Could you check a few things on this drawing? It's one solid part, dimensions in mm from its lowest x, y, z. A direction names the side the tool comes from. Round coordinates to 2 decimals unless told otherwise and drop trailing zeros. Write each loop counter-clockwise with the first axis right and the second up, starting at its lowest first coordinate (ties: lowest second). Pieces come first, ordered by that corner, then holes. Notation, with made-up numbers: (33.5, -24.75) -> (83.5, -24.75) arc R27 cw to (83.5, -2.75) -> close; hole circle Ø1 at (35, 57). An arc over 180 degrees is marked (long way). Return JSON: item names as keys, results as strings.
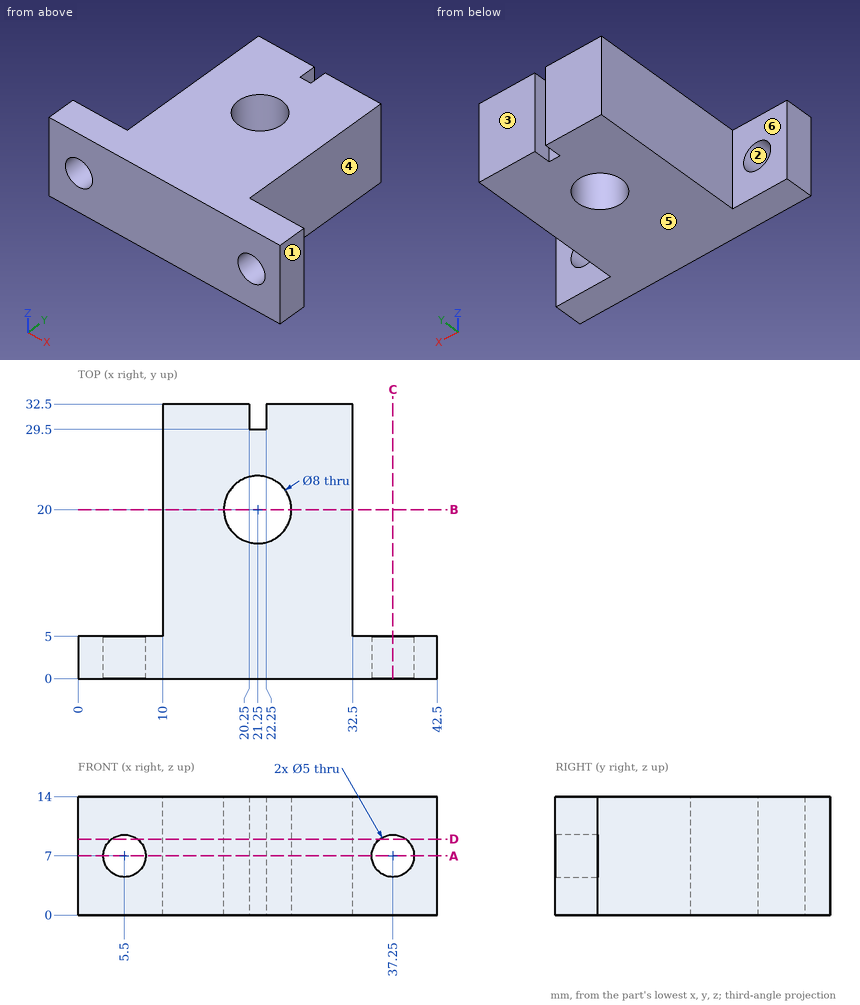
1) I want a section at A-A, the plane z = 7. Please give me the cut outline in (x, y), and give its area (3 significant figures).
Return value:
{"outline": "(0, 0) -> (3, 0) -> (3, 5) -> (0, 5) -> close; (8, 0) -> (34.75, 0) -> (34.75, 5) -> (32.5, 5) -> (32.5, 32.5) -> (22.25, 32.5) -> (22.25, 29.5) -> (20.25, 29.5) -> (20.25, 32.5) -> (10, 32.5) -> (10, 5) -> (8, 5) -> close; (39.75, 0) -> (42.5, 0) -> (42.5, 5) -> (39.75, 5) -> close; hole circle Ø8 at (21.25, 20)", "area": "725 mm²"}
2) Will these pins go through, and if not, where does the flat tip stop? pin 1 Ø3 at (y, z) = (21.5, 3) entering from -X; pin 2 Ø7 at (y, z) = (19.5, 7.5) entering from +X; pin 3 Ø5 at (x, z) = (4.5, 4.5) entering from +Y.
Return value:
{"pin 1": "x = 10", "pin 2": "x = 32.5", "pin 3": "y = 5"}
3) I want a section at D-D, the plane z = 9. Please give me the cut outline in (x, y).
Return value:
{"outline": "(0, 0) -> (4, 0) -> (4, 5) -> (0, 5) -> close; (7, 0) -> (35.75, 0) -> (35.75, 5) -> (32.5, 5) -> (32.5, 32.5) -> (22.25, 32.5) -> (22.25, 29.5) -> (20.25, 29.5) -> (20.25, 32.5) -> (10, 32.5) -> (10, 5) -> (7, 5) -> close; (38.75, 0) -> (42.5, 0) -> (42.5, 5) -> (38.75, 5) -> close; hole circle Ø8 at (21.25, 20)"}
4) I want a section at C-C, the plane x = 37.25. Please give me the cut outline in (y, z), and give its area (3 significant figures).
Return value:
{"outline": "(0, 0) -> (5, 0) -> (5, 4.5) -> (0, 4.5) -> close; (0, 9.5) -> (5, 9.5) -> (5, 14) -> (0, 14) -> close", "area": "45.0 mm²"}
5) Thinking about a two-plate mould opening in X: for the marked faces 1, 2 and 3, which applies, pulls with the +X half, pulls with the -X half, needs draft (parallel to the pull), parting line crosses it, or undercut?
Return value:
{"face 1": "pulls with the +X half", "face 2": "undercut", "face 3": "needs draft"}
6) For the marked faces 4, 5 and 6, which set-ups out of +Z, -Z, +X, -X, +Y, -Y let a thin tool reach every point of the face, with its end or its side?
Return value:
{"face 4": "+Z, -Z, +X, +Y", "face 5": "-Z, +X, -X, +Y, -Y", "face 6": "+Z, -Z, -X, +Y"}
7) I want a section at B-B, the plane y = 20. Please give me the cut outline in (x, z), and give its area (3 significant figures).
Return value:
{"outline": "(10, 0) -> (17.25, 0) -> (17.25, 14) -> (10, 14) -> close; (25.25, 0) -> (32.5, 0) -> (32.5, 14) -> (25.25, 14) -> close", "area": "203 mm²"}
8) If I drill on probe 1 along X at (y, z) = (31.5, 13); probe 2 along Y at (x, z) = (21.25, 8); probe 3 along Z at (x, y) = (37.25, 1.75), over which ranges is the centre line in solid material (lowest first)? Write a range as [from, to].
Return value:
{"probe 1": "[10, 20.25], [22.25, 32.5]", "probe 2": "[0, 16], [24, 29.5]", "probe 3": "[0, 4.5], [9.5, 14]"}
